from build123d import *

# Parameters (mm, degrees)
SKETCH1_R           = 4
SKETCH1_R_2         = 2.5
BOSS_EXTRUDE1_DEPTH = 1.25
SKETCH2_R           = 3.590807055
SKETCH2_R_2         = 2.909192945
CUT_EXTRUDE1_DEPTH  = 0.1


with BuildPart() as part:
    # Sketch1 → Boss-Extrude1 (new body)
    with BuildSketch(Plane(origin=(0, 0, 0), x_dir=(1, 0, 0), z_dir=(0, 1, 0))):
        with Locations(Location((0, 0, 0), (0, 0, 270))):
            Circle(SKETCH1_R)
        with Locations(Location((0, 0, 0), (0, 0, 270))):
            Circle(SKETCH1_R_2, mode=Mode.SUBTRACT)
    extrude(amount=BOSS_EXTRUDE1_DEPTH)

    # Sketch2 → Cut-Extrude1 (cut)
    with BuildSketch(Plane(origin=(0, 1.25, 0), x_dir=(1, 0, 0), z_dir=(0, 1, 0))):
        with Locations(Location((0, 0, 0), (0, 0, 270))):
            Circle(SKETCH2_R)
        with Locations(Location((0, 0, 0), (0, 0, 270))):
            Circle(SKETCH2_R_2, mode=Mode.SUBTRACT)
    extrude(amount=-CUT_EXTRUDE1_DEPTH, mode=Mode.SUBTRACT)

    # Mirror1: part across plane


with BuildPart() as part_1:
    add(part.part)
    add(part.part.mirror(Plane.ZX))


solid = part_1.part
Verification items for the finished model (mm, model axes). A direction names the side the tool comes from. Coordinates: 2 decimals unless noted, no trailing zeros. Order: outer loops, then holes, each group sorted by start corner. A loop starts at its lowest first (then second) coordinate and runs counter-clockwise, first axis right, second up. Notation, with made-up numbers: (0, -34) -> (34, -34) arc R33 cw to (34, -6) -> close; hole circle Ø9 at (27, 9.5). An arc over 180 degrees is marked (long way). Put each result on its own line as item: value. Start each with the question number.
1. Access from +Z, -Z, +X, -X, +Y, -Y to the whole of each face (thin tool, end or side, straight path). Record for faces 3 (the cylindrical face through (-2.44, -0.02, -0.54)), 4 (the flat face through (3, 1.15, -1)).
2. Material ranges on L1, parallel to X at y = -1.2, z = 0; L2, parallel to X at y = -0.4, z = 0; L3, parallel to X at y = -1.05, z = -1, recorded low to high. Write a range as [from, to].
3. Cross-section at A-A, the plane z = 0. Record the boundary of the cut face in (x, y), then the cut area to 3 significant figures.
4. Mould release check, pull along X, two halves, no side actions. Record for faces 1 (the cylindrical face through (-3.905, 0.018, -0.867)), 2 (the flat face through (3, -1.15, -1)): released by +X, released by -X, zero draft, split by the parting line, or undercut.
5. Cross-section at B-B, the plane x = 0. Record the boundary of the cut face in (y, z), then the cut area to 3 significant figures.
6. Cross-section at C-C, the plane y = -0.65. Record the boundary of the cut face in (x, z).
Computed:
1. face 3: +Y, -Y
1. face 4: +Y
2. L1: [-4, -3.59], [-2.91, -2.5], [2.5, 2.91], [3.59, 4]
2. L2: [-4, -2.5], [2.5, 4]
2. L3: [-3.87, -2.29], [2.29, 3.87]
3. outline: (-4, -1.25) -> (-3.59, -1.25) -> (-3.59, -1.15) -> (-2.91, -1.15) -> (-2.91, -1.25) -> (-2.5, -1.25) -> (-2.5, 1.25) -> (-2.91, 1.25) -> (-2.91, 1.15) -> (-3.59, 1.15) -> (-3.59, 1.25) -> (-4, 1.25) -> close; (2.5, -1.25) -> (2.91, -1.25) -> (2.91, -1.15) -> (3.59, -1.15) -> (3.59, -1.25) -> (4, -1.25) -> (4, 1.25) -> (3.59, 1.25) -> (3.59, 1.15) -> (2.91, 1.15) -> (2.91, 1.25) -> (2.5, 1.25) -> close
3. area: 7.23 mm2
4. face 1: split by the parting line
4. face 2: undercut
5. outline: (-1.25, -4) -> (1.25, -4) -> (1.25, -3.59) -> (1.15, -3.59) -> (1.15, -2.91) -> (1.25, -2.91) -> (1.25, -2.5) -> (-1.25, -2.5) -> (-1.25, -2.91) -> (-1.15, -2.91) -> (-1.15, -3.59) -> (-1.25, -3.59) -> close; (-1.25, 2.5) -> (1.25, 2.5) -> (1.25, 2.91) -> (1.15, 2.91) -> (1.15, 3.59) -> (1.25, 3.59) -> (1.25, 4) -> (-1.25, 4) -> (-1.25, 3.59) -> (-1.15, 3.59) -> (-1.15, 2.91) -> (-1.25, 2.91) -> close
5. area: 7.23 mm2
6. outline: circle Ø8 at (0, 0); hole circle Ø5 at (0, 0)
